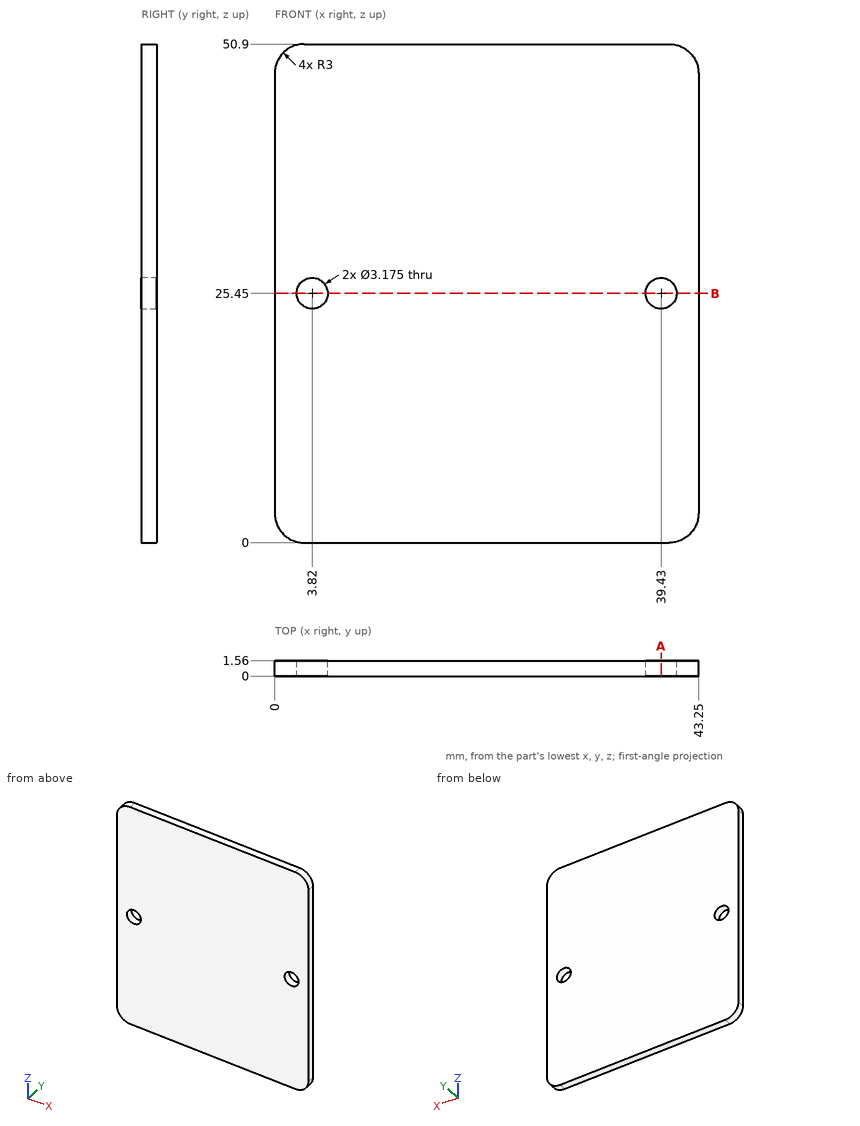
Verification items for this drawing (mm, ordinates from the low corner). Round coordinates to 2 decimals unless told otherwise and drop trailing zeros. Write each loop counter-clockwise with the first axis right and the second up, starting at its lowest first coordinate (ties: lowest second). Pieces come first, ordered by that corner, then holes. Notation, with made-up numbers: (-29.75, 47) - (-23.75, 47) arc R18 cw to (-23.75, 65) - close; hole circle Ø6 at (81.5, 64). An arc over 180 degrees is marked (long way). Answer as a JSON object with one key per item and string values. Group by question number.
Q1. Thickness scan on line 1 (X direction, y = 1.2, z = 25.45); line 2 (Z direction, x = 39.5, y = 0.65). Record the ranges inside material, lowest first.
Q2. Section check A-A, the plane x = 39.43. Enter the section's corners in (y, z), plus the area to 3 significant figures.
Q3. Section check B-B, the plane z = 25.45. Enter the section's corners in (x, y).
Found:
{
 "1": {"line 1": "x = 0 to 2.23, 5.41 to 37.84, 41.02 to 43.25", "line 2": "z = 0 to 23.86, 27.04 to 50.9"},
 "2": {"outline": "(0, 0) - (1.56, 0) - (1.56, 23.86) - (0, 23.86) - close; (0, 27.04) - (1.56, 27.04) - (1.56, 50.9) - (0, 50.9) - close", "area": "74.5 mm^2"},
 "3": {"outline": "(0, 0) - (2.23, 0) - (2.23, 1.56) - (0, 1.56) - close; (5.41, 0) - (37.84, 0) - (37.84, 1.56) - (5.41, 1.56) - close; (41.02, 0) - (43.25, 0) - (43.25, 1.56) - (41.02, 1.56) - close"}
}
